Here's the drawing with two shaded views (mm, measured from the low corner). I have some questions. A direction names the side the tool comes from. Give positions to 0.01 mm unless a question says otherwise; leave off trailing zeros. Loops run counter-clockwise (first coordinate to the right, second up) from the corner with the lowest first, then second, coordinate; pieces in that order, holes last. Notation, with made-up numbers: (36, 17) -> (52, 17) arc R15 ccw to (52, 33) -> close; hole circle Ø2 at (36.25, 32.5). An arc over 180 degrees is marked (long way). Put each result on its own line as item: value.
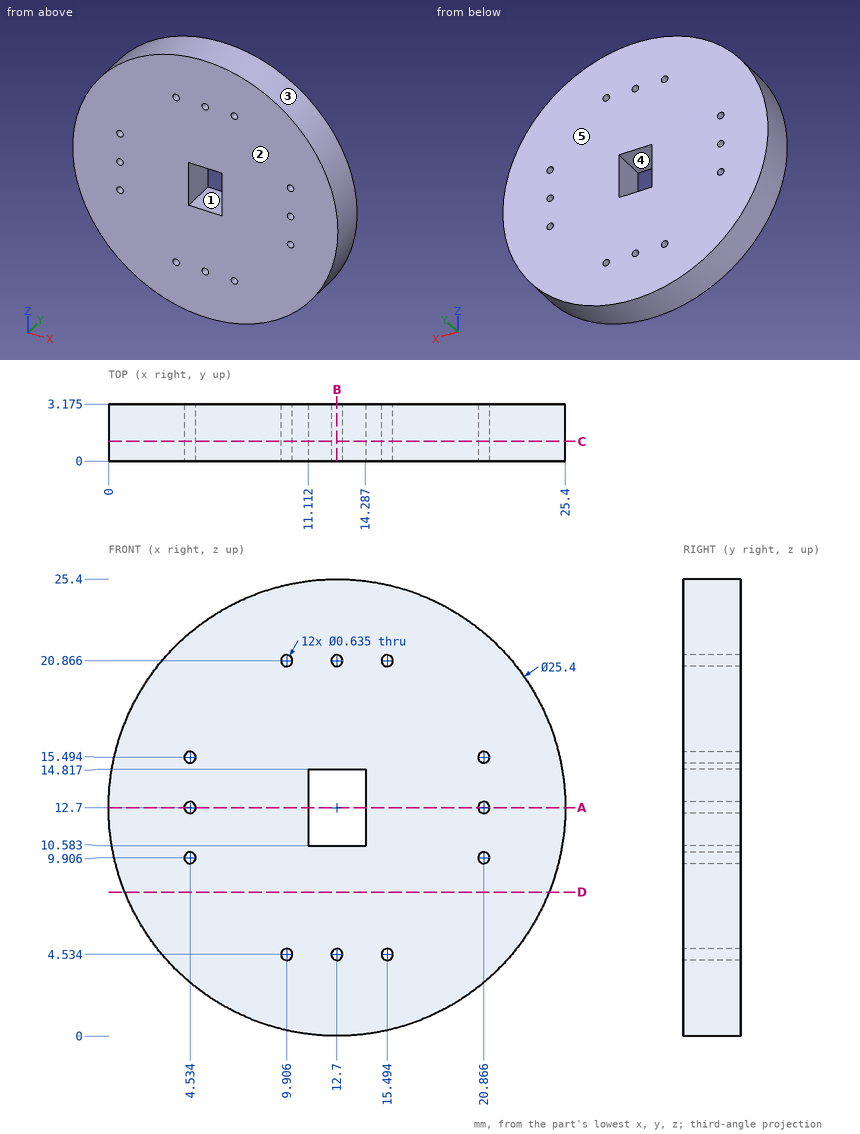
1. If we section it at A-A (z = 12.7): List the corners of the cut face in (x, y) for me (1 decimal).
Recorded:
outline: (0, 0) -> (4.2, 0) -> (4.2, 3.2) -> (0, 3.2) -> close; (4.9, 0) -> (11.1, 0) -> (11.1, 3.2) -> (4.9, 3.2) -> close; (14.3, 0) -> (20.5, 0) -> (20.5, 3.2) -> (14.3, 3.2) -> close; (21.2, 0) -> (25.4, 0) -> (25.4, 3.2) -> (21.2, 3.2) -> close
2. If we section it at B-B (x = 12.7): List the corners of the cut face in (y, z) for me (1 decimal).
Recorded:
outline: (0, 0) -> (3.2, 0) -> (3.2, 4.2) -> (0, 4.2) -> close; (0, 4.9) -> (3.2, 4.9) -> (3.2, 10.6) -> (0, 10.6) -> close; (0, 14.8) -> (3.2, 14.8) -> (3.2, 20.5) -> (0, 20.5) -> close; (0, 21.2) -> (3.2, 21.2) -> (3.2, 25.4) -> (0, 25.4) -> close
3. Thinking about a two-plate mould opening in Z: for the marked faces 1, 2 and 3, which applies, pulls with the +Z half, pulls with the -Z half, needs draft (parallel to the pull), parting line crosses it, or undercut?
Recorded:
face 1: undercut
face 2: needs draft
face 3: parting line crosses it
4. If we section it at D-D (z = 8): List the corners of the cut face in (x, y) for me (1 decimal).
Recorded:
outline: (0.9, 0) -> (24.5, 0) -> (24.5, 3.2) -> (0.9, 3.2) -> close
5. I'm going to push flat-ended pins straight in: pin 1 (5 mm diameter, centred on x = 6.5, z = 16, fed in from -Y); pin 2 (1.5 mm diameter, centred on x = 17.5, y = 2, fed in from -Z). Where does each tip first touch, or does it pass through?
Recorded:
pin 1: stops at y = 0
pin 2: stops at z = 0.66
6. I need wall thicknesses on line 1 (Z direction, x = 12.7, y = 1.85); line 2 (X direction, y = 0.5, z = 10); line 3 (X direction, y = 0.2, z = 13.25). Which ranges of each line are inside material? Lowest first, please.
Recorded:
line 1: z = 0 to 4.22, 4.85 to 10.58, 14.82 to 20.55, 21.18 to 25.4
line 2: x = 0.29 to 4.23, 4.84 to 20.56, 21.17 to 25.11
line 3: x = 0.01 to 11.11, 14.29 to 25.39
7. For the marked faces 4 and 5, which set-ups out of +Z, -Z, +X, -X, +Y, -Y let a thin tool reach every point of the face, with its end or its side?
Recorded:
face 4: +Y, -Y
face 5: +Z, -Z, +X, -X, +Y
8. If we section it at C-C (y = 1.1): Count the separate pieces of the cut face and the enclosed holes in it.
Recorded:
separate pieces: 1
enclosed holes: 13
